```python
from build123d import *

# Parameters (mm, degrees)
F0_R     = 3.5
F1_DEPTH = 3
F2_R     = 0.5
F3_R     = 0.5


with BuildPart() as f1:
    # F0 (on Top) → F1 (new body)
    with BuildSketch(Plane.XY):
        Polygon((5.5, -3.175426), (5.5, 3.175426), (0, 6.350853), (-5.5, 3.175426), (-5.5, -3.175426), (0, -6.350853), align=None)
        Circle(F0_R, mode=Mode.SUBTRACT)
    extrude(amount=F1_DEPTH)

    # F2
    f2_edges = [f1.edges().sort_by_distance(p)[0] for p in [
        (2.75, -4.76314, 3),
        (-2.75, -4.76314, 3),
        (-2.75, 4.76314, 3),
        (-5.5, 0, 3),
        (5.5, 0, 3),
        (2.75, 4.76314, 3),
    ]]
    fillet(f2_edges, radius=F2_R)

    # F3
    f3_edges = [f1.edges().sort_by_distance(p)[0] for p in [
        (2.75, -4.76314, 0),
        (-2.75, -4.76314, 0),
        (-2.75, 4.76314, 0),
        (-5.5, 0, 0),
        (2.75, 4.76314, 0),
        (5.5, 0, 0),
    ]]
    fillet(f3_edges, radius=F3_R)


solid = f1.part
```
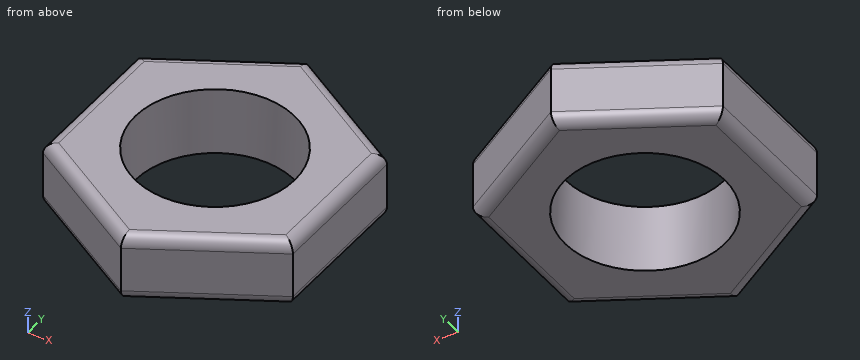
Geometry: final body of the model. Coordinates: model frame, mm. Round coordinates to 2 decimals unless told otherwise and drop trailing zeros. Write each loop counter-clockwise with the first axis right and the second up, starting at its lowest first coordinate (ties: lowest second). Pieces come first, ordered by that corner, then holes.
Item 1: Pin query (flat end, axial travel): P1, Ø1.5, axis at x = 3.5, z = 2.5, coming from the +Y side; P2, Ø1, axis at x = -1, y = -2, coming from the +Z side. Return the tip coordinate at first contact, or that it passes through.
Item 2: Section query A-A (y = 0). Return loops of the section in (x, z).
Item 3: Section query B-B (z = 2.1). Return loops of the section in (x, y), plus the area to 3 significant figures.
Item 4: Material intervals for L1, parallel to Y at x = 1.5, z = 1.9; L2, parallel to Y at x = 1, z = 0.3; L3, parallel to X at y = 1, z = 0.75, sorted ascending.
Completed:
1. P1: stops at y = 4.76
1. P2: passes through
2. outline: (-5.5, 0.5) arc R0.5 ccw to (-5, 0) - (-3.5, 0) - (-3.5, 3) - (-5, 3) arc R0.5 ccw to (-5.5, 2.5) - close; (3.5, 0) - (5, 0) arc R0.5 ccw to (5.5, 0.5) - (5.5, 2.5) arc R0.5 ccw to (5, 3) - (3.5, 3) - close
3. outline: (-5.5, -3.18) - (0, -6.35) - (5.5, -3.18) - (5.5, 3.18) - (0, 6.35) - (-5.5, 3.18) - close; hole circle Ø7 at (0, 0)
3. area: 66.3 mm2
4. L1: y = -5.48 to -3.16, 3.16 to 5.48
4. L2: y = -5.73 to -3.35, 3.35 to 5.73
4. L3: x = -5.5 to -3.35, 3.35 to 5.5
